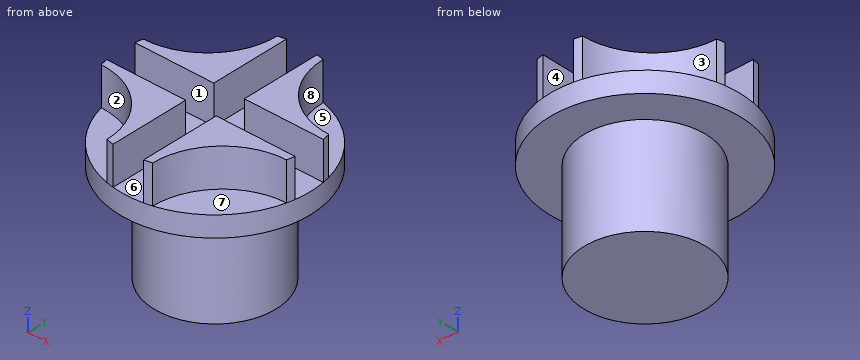
```python
from build123d import *

# Parameters (mm, degrees)
CROQUIS1_R              = 12.5
SALIENTE_EXTRUIR1_DEPTH = 2.7
SALIENTE_EXTRUIR2_START = 2.7
SALIENTE_EXTRUIR2_DEPTH = 5
CROQUIS2_R              = 8
SALIENTE_EXTRUIR3_DEPTH = 13


with BuildPart() as part:
    # Croquis1 → Saliente-Extruir1 (new body)
    with BuildSketch(Plane.XY):
        Circle(CROQUIS1_R)
    extrude(amount=SALIENTE_EXTRUIR1_DEPTH)

    # Croquis1<3> → Saliente-Extruir2 (add)
    with BuildSketch(Plane.XY.offset(SALIENTE_EXTRUIR2_START)):
        with BuildLine():
            Line((-2, 2), (-2, 12.338962679))
            ThreePointArc((-2, 12.338962679), (-2.502086086, 12.247022708), (-3, 12.1346611))
            ThreePointArc((-3, 12.1346611), (-5.694387223, 5.694387223), (-12.1346611, 3))
            ThreePointArc((-12.1346611, 3), (-12.247022708, 2.502086086), (-12.338962679, 2))
            Line((-12.338962679, 2), (-2, 2))
        make_face()
        with BuildLine():
            ThreePointArc((3, 12.1346611), (2.502086086, 12.247022708), (2, 12.338962679))
            Line((2, 12.338962679), (2, 2))
            Line((2, 2), (12.338962679, 2))
            ThreePointArc((12.338962679, 2), (12.247022708, 2.502086086), (12.1346611, 3))
            ThreePointArc((12.1346611, 3), (5.694387223, 5.694387223), (3, 12.1346611))
        make_face()
        with BuildLine():
            Line((12.338962679, -2), (2, -2))
            Line((2, -2), (2, -12.338962679))
            ThreePointArc((2, -12.338962679), (2.502086086, -12.247022708), (3, -12.1346611))
            ThreePointArc((3, -12.1346611), (5.694387223, -5.694387223), (12.1346611, -3))
            ThreePointArc((12.1346611, -3), (12.247022708, -2.502086086), (12.338962679, -2))
        make_face()
        with BuildLine():
            Line((-2, -12.338962679), (-2, -2))
            Line((-2, -2), (-12.338962679, -2))
            ThreePointArc((-12.338962679, -2), (-12.247022708, -2.502086086), (-12.1346611, -3))
            ThreePointArc((-12.1346611, -3), (-5.694387223, -5.694387223), (-3, -12.1346611))
            ThreePointArc((-3, -12.1346611), (-2.502086086, -12.247022708), (-2, -12.338962679))
        make_face()
    extrude(amount=SALIENTE_EXTRUIR2_DEPTH)

    # Croquis2 → Saliente-Extruir3 (add)
    with BuildSketch(Plane(origin=(0, 0, 0), x_dir=(-1, 0, 0), z_dir=(0, 0, -1))):
        Circle(CROQUIS2_R)
    extrude(amount=SALIENTE_EXTRUIR3_DEPTH)


solid = part.part
```
Model file for the job. Use its own axes, mm. Face numbers are marked on the shaded views. A direction names the side the tool comes from. Give positions to 0.01 mm unless a question says otherwise; leave off trailing zeros. Loops run counter-clockwise (first coordinate to the right, second up) from the corner with the lowest first, then second, coordinate; pieces in that order, holes last. Notation, with made-up numbers: M 39,-24 L 50,-24 A22 ccw 50,-16 Z; hole C 57,10.25 d10. An arc over 180 degrees is marked long. Use one line per item in the form item = value.
Item 1: Drill centre lines: L1, parallel to Z at x = -8.5, y = -6.75; L2, parallel to Z at x = 1.5, y = -4.25; L3, parallel to Y at x = -11.5, z = 4. Where is each one in solid material? Low to high.
Filled in:
L1 = 0 to 2.7
L2 = -13 to 2.7
L3 = -3.03 to -2, 2 to 3.03
Item 2: Slice it at C-C on z = -9. List the corners of the cut face in (x, y), and give its area (3 significant figures).
Filled in:
outline = C 0,0 d16
area = 201 mm^2
Item 3: Slice it at D-D on x = -2.5. List the corners of the cut face in (y, z), and give its area (3 significant figures).
Filled in:
outline = M -12.25,0 L -7.6,0 L -7.6,-13 L 7.6,-13 L 7.6,0 L 12.25,0 L 12.25,7.7 L 2,7.7 L 2,2.7 L -2,2.7 L -2,7.7 L -12.25,7.7 Z
area = 366 mm^2
Item 4: Flat gauge pins, fed straight in: pin 1 Ø1.5 at (y, z) = (9, 5.5) entering from -X; pin 2 Ø4.5 at (x, y) = (-8, -9.5) entering from +Z; pin 3 Ø4 at (x, z) = (7, 4.5) entering from -Y. Where does each tip first touch, or does it go through?
Filled in:
pin_1 = -3.89
pin_2 = 2.7
pin_3 = -10.89
Item 5: Two-plate mould, pull along X, no slides. Class the marked faces 6, 7 and 8: released by +X, released by -X, zero draft, split by the parting line, or undercut.
Filled in:
face_6 = undercut
face_7 = zero draft
face_8 = released by +X
Item 6: Slice it at A-A on x = 0. List the corners of the cut face in (y, z), and give its area (4 significant figures).
Filled in:
outline = M -12.5,0 L -8,0 L -8,-13 L 8,-13 L 8,0 L 12.5,0 L 12.5,2.7 L -12.5,2.7 Z
area = 275.5 mm^2
Item 7: Slice it at B-B on y = 5.25. List the corners of the cut face in (x, z), and give its area (3 significant figures).
Filled in:
outline = M -11.34,0 L -6.04,0 L -6.04,-13 L 6.04,-13 L 6.04,0 L 11.34,0 L 11.34,2.7 L 6.17,2.7 L 6.17,7.7 L 2,7.7 L 2,2.7 L -2,2.7 L -2,7.7 L -6.17,7.7 L -6.17,2.7 L -11.34,2.7 Z
area = 260 mm^2
Item 8: Which spindle directions (+Z, -Z, +X, -X, +Y, -Y) get a long thin tool onto all of the face, cutting with end or side? Do the marked faces 1, 2, 3, 4 and 5. Say none if no direction does.
Filled in:
face_1 = +Z, +X, -X
face_2 = +Z, -X, -Y
face_3 = +Z, -X, +Y
face_4 = +Z, +Y, -Y
face_5 = +Z, +X, +Y
